The listing builds one solid part. Answer for the finished solid, in the listing's coordinates (mm). A direction names the side the tool comes from. Coordinates: 2 decimals unless noted, no trailing zeros. Order: outer loops, then holes, each group sorted by start corner. A loop starts at its lowest first (then second) coordinate and runs counter-clockwise, first axis right, second up.
```python
from build123d import *

# Parameters (mm, degrees)
CHAMFER_1_SIZE  = 0.26
CHAMFER_1_SIZE2 = 3


with BuildPart() as part:
    # Эскиз1 → Повернуть1 (revolve)
    with BuildSketch(Plane.XY):
        Polygon((0, 0), (0, 21.5), (-4.5, 21.5), (-4.5, 1.5), (-9, 1.5), (-9, -2), (-8, -2), (-8, 0), align=None)
    revolve(axis=Axis((0, 0, 0), (0, 1, 0)))

    # Фаска1
    chamfer_1_edges = [part.edges().sort_by_distance(p)[0] for p in [
        (4.5, 21.5, 0),
    ]]
    chamfer_1_side = [part.faces().sort_by_distance(p)[0] for p in [
        (0, 21.5, 0),
    ]]
    chamfer(chamfer_1_edges, length=CHAMFER_1_SIZE, length2=CHAMFER_1_SIZE2, reference=chamfer_1_side[0])


solid = part.part
```
1) Straight lines are drawn through the part: probe 1 along Z at (x, y) = (0, -1.25); probe 2 along Y at (x, z) = (0.75, -4); probe 3 along Z at (x, y) = (1.5, 14). For each, find the intervals that lie inside material, in ascending order.
2) For faces 1 (the cylindrical face through (0.59, 9.88, 4.46)), 2 (the flat face through (0, 0, 0)), 3 (the flat face through (0, 21.5, 0)), determine the directions among +Z, -Z, +X, -X, +Y, -Y from which every point of the face is accessible in a straight line to the end or side of a thin tool.
3) A cutting plane is placed at B-B, the plane z = 0. Write down the section's boundary in (x, y).
4) A cutting plane is placed at D-D, the plane x = -6.5. Write down the section's boundary in (y, z).
5) A cutting plane is placed at A-A, the plane x = 0. Write down the section's boundary in (y, z).
6) Each of these flat-tipped pins is pushed along its axis until it touches: P1, Ø2, axis at x = 6, z = 5.5, coming from the +Y side; P2, Ø5, axis at x = 2, y = 17.5, coming from the +Z side; P3, Ø1, axis at x = 0, z = 3, coming from the -Y side. Where does it stop, or does it pass through?
7) The mould has two halves that part along Z. Classify faces 4 (the flat face through (4, 1.5, -4)), 5 (the cylindrical face through (1.73, -0.99, -7.81)), 6 (the cylindrical face through (1.172, -0.274, 8.923)): released by +Z, released by -Z, zero draft, split by the parting line, or undercut.
8) A cutting plane is placed at C-C, the plane y = 9.75. Write down the section's boundary in (x, z), plus the area to 3 significant figures.
Working result:
1. probe 1: z = -9 to -8, 8 to 9
1. probe 2: y = 0 to 21.5
1. probe 3: z = -4.24 to 4.24
2. face 1: +Y
2. face 2: -Y
2. face 3: +Z, -Z, +X, -X, +Y
3. outline: (-9, -2) - (-8, -2) - (-8, 0) - (8, 0) - (8, -2) - (9, -2) - (9, 1.5) - (4.5, 1.5) - (4.5, 18.5) - (4.24, 21.5) - (-4.24, 21.5) - (-4.5, 18.5) - (-4.5, 1.5) - (-9, 1.5) - close
4. outline: (-2, -6.22) - (1.5, -6.22) - (1.5, 6.22) - (-2, 6.22) - (-2, 4.66) - (0, 4.66) - (0, -4.66) - (-2, -4.66) - close
5. outline: (-2, -9) - (1.5, -9) - (1.5, -4.5) - (18.5, -4.5) - (21.5, -4.24) - (21.5, 4.24) - (18.5, 4.5) - (1.5, 4.5) - (1.5, 9) - (-2, 9) - (-2, 8) - (0, 8) - (0, -8) - (-2, -8) - close
6. P1: stops at y = 1.5
6. P2: stops at z = 4.5
6. P3: stops at y = 0
7. face 4: zero draft
7. face 5: undercut
7. face 6: split by the parting line
8. outline: circle Ø9 at (0, 0)
8. area: 63.6 mm2
